```python
from build123d import *

# Parameters (mm, degrees)
F0_R     = 38.1
F0_R_2   = 19.5559303257
F1_DEPTH = 25.4
F2_W     = 25.4
F2_H     = 8.8900010133
F3_ANGLE = 180
F4_R     = 3.81
F5_SIZE  = 3.81


with BuildPart() as f1:
    # F0 (on Front) → F1 (new body)
    with BuildSketch(Plane.XZ):
        Circle(F0_R)
        Circle(F0_R_2, mode=Mode.SUBTRACT)
    extrude(amount=F1_DEPTH)

    # F2 (on face) → F3 (revolve)
    with BuildSketch(Plane.XZ.offset(25.4)):
        with Locations((0, 27.3050005066)):
            Rectangle(F2_W, F2_H)
    revolve(axis=Axis((9.351817891, -25.4, 0), (1, 0, 0)), revolution_arc=F3_ANGLE)

    # F4
    f4_edges = [f1.edges().sort_by_distance(p)[0] for p in [
        (-12.7, -57.150001, 0),
        (12.7, -57.150001, 0),
        (12.7, -48.26, 0),
        (-12.7, -48.26, 0),
    ]]
    fillet(f4_edges, radius=F4_R)

    # F5
    f5_edges = [f1.edges().sort_by_distance(p)[0] for p in [
        (38.1, -12.7, 0),
        (-38.1, 0, 0),
        (-38.1, -25.4, 0),
    ]]
    chamfer(f5_edges, length=F5_SIZE)


solid = f1.part
```
Can you work these out from the model? Positions are in its coordinate system, mm. A direction names the side the tool comes from. Coordinates: 2 decimals unless noted, no trailing zeros. Loops run counter-clockwise (first coordinate to the right, second up) from the corner with the lowest first, then second, coordinate; pieces in that order, holes last.
1) Thinking about a two-plate mould opening in Z: for faces 6 (the cylindrical face through (0.124, -48.254, 0.503)), 7 (the flat face through (15, 0, -15)), 8 (the cylindrical face through (0.124, -57.142, 0.698)), which applies, pulls with the +Z half, pulls with the -Z half, needs draft (parallel to the pull), parting line crosses it, or undercut?
2) For pin 1 (6 mm diameter, centred on x = -14, y = -31, fed in from -Z); pin 2 (14 mm diameter, centred on y = -46, z = -2, fed in from +X); pin 3 (1 mm diameter, centred on x = 12, y = -27.5, fed in from +Z); pin 4 (1.5 mm diameter, centred on x = -25, z = 30.5, fed in from +Y), each with a flat end and sliding along its axis, tell me the tip position at first contact or that it passes through.
3) Imagine slicing it at A-A on z = 0. List the corners of the cut face in (x, y) for me.
4) Which directions (+Z, -Z, +X, -X, +Y, -Y) give clear straight access to the entire face, cutting with the end or side of a thin tool? Please do faces 1 (the flat face through (-12.7, -52, 4)), 2 (the cylindrical face through (18.653, -12.522, 5.874)), 3 (the cylindrical face through (-30.235, -12.576, -23.183)), 4 (the flat face through (12.7, -52, 4)), 5 (the conical face through (-7.49, -25.16, -33.71)).
5) Imagine slicing it at B-B on x = 0. List the corners of the cut face in (y, z) for me.
6) I need wall thicknesses on probe 1 along Z at (x, y) = (0, -10); probe 2 along Y at (x, z) = (-27, 18); probe 3 along Z at (x, y) = (4, -5). Which ranges of each line are inside material? Lowest first, please.
7) Imagine slicing it at C-C on y = -15. List the corners of the cut face in (x, z) for me, plus the area to 3 significant figures.
Completed:
1. face 6: undercut
1. face 7: needs draft
1. face 8: parting line crosses it
2. pin 1: stops at z = -30.67
2. pin 2: stops at x = 12.7
2. pin 3: stops at z = 30.64
2. pin 4: passes through
3. outline: (-38.1, -21.59) - (-34.29, -25.4) - (-19.56, -25.4) - (-19.56, 0) - (-34.29, 0) - (-38.1, -3.81) - close; (-12.7, -53.34) arc R3.81 ccw to (-8.89, -57.15) - (8.89, -57.15) arc R3.81 ccw to (12.7, -53.34) - (12.7, -52.07) arc R3.81 ccw to (8.89, -48.26) - (-8.89, -48.26) arc R3.81 ccw to (-12.7, -52.07) - close; (19.56, -25.4) - (34.29, -25.4) - (38.1, -21.59) - (38.1, -3.81) - (34.29, 0) - (19.56, 0) - close
4. face 1: +Z, -Z, -X, -Y
4. face 2: +Y
4. face 3: +Y, -Y
4. face 4: +Z, -Z, +X, -Y
4. face 5: -Y
5. outline: (-25.4, -34.29) - (-21.59, -38.1) - (-3.81, -38.1) - (0, -34.29) - (0, -19.56) - (-25.4, -19.56) - (-25.4, -22.86) arc R22.86 cw to (-25.4, 22.86) - (-25.4, 19.56) - (0, 19.56) - (0, 34.29) - (-3.81, 38.1) - (-21.59, 38.1) - (-25.4, 34.29) - (-25.4, 31.75) arc R31.75 ccw to (-25.4, -31.75) - close
6. probe 1: z = -38.1 to -19.56, 19.56 to 38.1
6. probe 2: y = -25.4 to 0
6. probe 3: z = -37.89 to -19.14, 19.14 to 37.89
7. outline: circle Ø76.2 at (0, 0); hole circle Ø39.11 at (0, 0)
7. area: 3,360 mm2
